Geometry check sheet. Reference: the model listing, model coordinates, mm. A direction names the side the tool comes from. Round coordinates to 2 decimals unless told otherwise and drop trailing zeros. Loops run counter-clockwise (first coordinate to the right, second up) from the corner with the lowest first, then second, coordinate; pieces in that order, holes last. Notation, with made-up numbers: M -31.5,-24 L 24.5,-24 A9 ccw 24.5,-14 Z; hole C 54,22 d10. An arc over 180 degrees is marked long. Answer in a Markdown table with one row per item. Add a question column.
```python
from build123d import *

# Parameters (mm, degrees)
SKETCH2_W           = 57.15
SKETCH2_H           = 25.4
BOSS_EXTRUDE1_DEPTH = 3.175
HOLE1_D             = 6.35
CHAMFER1_SIZE       = 7.62
CUT_EXTRUDE1_DEPTH  = 32.430896424


with BuildPart() as part:
    # Sketch2 → Boss-Extrude1 (new body)
    with BuildSketch(Plane.XY):
        Rectangle(SKETCH2_W, SKETCH2_H)
    extrude(amount=BOSS_EXTRUDE1_DEPTH)

    # Hole1 (through all)
    with Locations(Plane.XY.offset(3.175)):
        with Locations((-19.05, 0), (19.05, 0)):
            Hole(HOLE1_D / 2)

    # Chamfer1
    chamfer1_edges = [part.edges().sort_by_distance(p)[0] for p in [
        (28.575, -12.7, 1.5875),
        (-28.575, -12.7, 1.5875),
        (-28.575, 12.7, 1.5875),
        (28.575, 12.7, 1.5875),
    ]]
    chamfer(chamfer1_edges, length=CHAMFER1_SIZE)

    # Sketch5 → Cut-Extrude1 (cut, through all)
    with BuildSketch(Plane.XY.offset(3.175)):
        Polygon((7.62, 3.156307345), (3.156307345, 7.62), (-3.156307345, 7.62), (-7.62, 3.156307345), (-7.62, -3.156307345), (-3.156307345, -7.62), (3.156307345, -7.62), (7.62, -3.156307345), align=None)
    extrude(amount=-CUT_EXTRUDE1_DEPTH, mode=Mode.SUBTRACT)


solid = part.part
```
1) Cross-section at D-D, the plane y = 10. Record the boundary of the cut face in (x, z) (3 decimals).
2) Cross-section at C-C, the plane y = 0. Record the boundary of the cut face in (x, z) (3 decimals).
3) Set-up check for faces 5 (the flat face through (-24.712, -8.943, 1.565)), 6 (the flat face through (-5.419, -5.357, 1.61)): record each of +Z, -Z, +X, -X, +Y, -Y from which the full face is reachable in a straight line by a thin tool's end or side.
4) Go/stop test with a flat-tipped pin: pin 1 (4 mm diameter, centred on x = -19.05, y = 0, fed in from +Z). Record where the tip stops, or that it passes through.
5) Draft check along Y on faces 1 (the flat face through (5.357, -5.419, 1.61)), 2 (the flat face through (7.62, 0, 2)), 3 (the flat face through (24.818, 8.837, 1.565)), 4 (the flat face through (-28.575, 0, 2)). Enter one of: +Y half, -Y half, draft (parallel to the pull), parting line (faces both ways), or undercut.
6) Cross-section at A-A, the plane x = -19.05. Record the boundary of the cut face in (y, z) (3 decimals).
7) Thickness scan on L1, parallel to Y at x = 2, z = 1.7; L2, parallel to Y at x = -19.05, z = 0.95 (3 decimals); L3, parallel to X at y = 3.75, z = 1.4 (3 decimals). Record the ranges inside material, lowest first. Write a range as [from, to].
8) Cross-section at B-B, the plane z = 1.2. Record the boundary of the cut face in (x, y) (3 decimals).
Worked answers:
| question | item | result |
|---|---|---|
| 1 | outline | M -23.655,0 L 23.655,0 L 23.655,3.175 L -23.655,3.175 Z |
| 2 | outline | M -28.575,0 L -22.225,0 L -22.225,3.175 L -28.575,3.175 Z; M -15.875,0 L -7.62,0 L -7.62,3.175 L -15.875,3.175 Z; M 7.62,0 L 15.875,0 L 15.875,3.175 L 7.62,3.175 Z; M 22.225,0 L 28.575,0 L 28.575,3.175 L 22.225,3.175 Z |
| 3 | face 5 | +Z, -Z, -X, -Y |
| 3 | face 6 | +Z, -Z |
| 4 | pin 1 | passes through |
| 5 | face 1 | undercut |
| 5 | face 2 | undercut |
| 5 | face 3 | +Y half |
| 5 | face 4 | draft |
| 6 | outline | M -12.7,0 L -3.175,0 L -3.175,3.175 L -12.7,3.175 Z; M 3.175,0 L 12.7,0 L 12.7,3.175 L 3.175,3.175 Z |
| 7 | L1 | y = [-12.7, -7.62], [7.62, 12.7] |
| 7 | L2 | y = [-12.7, -3.175], [3.175, 12.7] |
| 7 | L3 | x = [-28.575, -7.026], [7.026, 28.575] |
| 8 | outline | M -28.575,-5.08 L -20.955,-12.7 L 20.955,-12.7 L 28.575,-5.08 L 28.575,5.08 L 20.955,12.7 L -20.955,12.7 L -28.575,5.08 Z; hole C -19.05,0 d6.35; hole M -7.62,-3.156 L -3.156,-7.62 L 3.156,-7.62 L 7.62,-3.156 L 7.62,3.156 L 3.156,7.62 L -3.156,7.62 L -7.62,3.156 Z; hole C 19.05,0 d6.35 |
